Read the model definition and answer for the solid it produces. Units are mm, in the model's axes. A direction names the side the tool comes from. Give positions to 0.01 mm unless a question says otherwise; leave off trailing zeros. Order: outer loops, then holes, each group sorted by start corner. A loop starts at its lowest first (then second) coordinate and runs counter-clockwise, first axis right, second up. Notation, with made-up numbers: (3.5, -5.75) - (41.5, -5.75) arc R15 ccw to (41.5, 9.25) - close; hole circle Ø8 at (67.5, 11). An arc over 180 degrees is marked (long way). Write each question's results on one line, items separated by ' | '. Start each with the question number.
Q1. Find the intervals of material crossed by line 1 along Z through (x, y) = (67, 27); line 2 along Z through (x, y) = (10.5, 12); line 3 along X through (y, z) = (34, 91), in increasing order. Write a range as from..to.
Q2. Flat-ended cylindrical pins translate along their axes: P1, Ø10, axis at y = 9, z = 24, coming from the +X side; P2, Ø6, axis at x = 21, y = 24.5, coming from the -Z side; P3, Ø22.5, axis at x = 49.5, z = 61.5, coming from the -Y side; P4, Ø0.5, axis at y = 20.5, z = 77, coming from the -X side. Find the tip coordinate at first contact, or state that the pin passes through.
Q3. A tool of negligible diameter and unlimited length cuts with its end or side. For faces 4 (the face through (4.88, 33.17, 80.28)), 5 (the face through (38, 36, 15)), 6 (the face through (57.2, 20, 60.4)), 7 (the face through (67, 25, 60)), from which of +Z, -Z, +X, -X, +Y, -Y can it reach the whole face along a straight path? Write none if from no direction.
Q4. Find section C-C on z = 39.5. Give the vertices of the cut face in (x, y) (3 decimals).
Q5. For a pull along X with two mould halves and no side action, classify faces 1 (the face through (17, 0, 30)), 2 (the face through (90.14, 32.675, 50.7)), 3 (the face through (17, 23, 60)) as +X half, -X half, draft (parallel to the pull), parting line (faces both ways), or undercut.
Q6. Find section B-B on x = 71. Give the vertices of the cut face in (y, z).
Q7. Find section D-D on y = 31.5. Give the vertices of the cut face in (x, z).
Q8. Find section A-A on z = 80. Give the vertices of the cut face in (x, y) (3 decimals).
from build123d import *

# Parameters (mm, degrees)
F0_W     = 65
F0_H     = 25
F1_DEPTH = 100
F4_DEPTH = 40
F5_DEPTH = 85
F6_W     = 10
F6_H     = 30
F7_DEPTH = 55
F9_DEPTH = 100.001


with BuildPart() as f1:
    # F0 (on Top) → F1 (new body)
    with BuildSketch(Plane.XY):
        Polygon((0, 45), (0, 0), (35, 0), (35, 20), (35, 45), align=None)
        with Locations((67.5, 32.5)):
            Rectangle(F0_W, F0_H)
    extrude(amount=F1_DEPTH)

    # F2 (on face) → F4 (cut, through all)
    with BuildSketch(Plane.XY.offset(100)):
        Polygon((35, 0), (35, 20), (35, 21), (35, 45), (9.6249980852, 45), (0, 21), (0, 0), align=None)
    extrude(amount=-F4_DEPTH, mode=Mode.SUBTRACT)

    # F2 (on face) → F5 (cut)
    with BuildSketch(Plane.XY.offset(100)):
        Polygon((35, 45), (35, 21), (44.124994427, 45), align=None)
    extrude(amount=-F5_DEPTH, mode=Mode.SUBTRACT)

    # F6 (on face) → F7 (cut)
    with BuildSketch(Plane.YZ.offset(100)):
        with Locations((25, 45)):
            Rectangle(F6_W, F6_H)
    extrude(amount=-F7_DEPTH, mode=Mode.SUBTRACT)

    # F8 (on face) → F9 (cut, through all)
    with BuildSketch(Plane.XY.offset(100)):
        Polygon((100, 20), (100, 45), (80, 20), align=None)
    extrude(amount=-F9_DEPTH, mode=Mode.SUBTRACT)


solid = f1.part
Working result:
1) line 1: 0..30, 60..100 | line 2: 0..60 | line 3: 0..5.21, 39.94..91.2
2) P1: x = 35 | P2: z = 0 | P3: y = 20 | P4: x = 35
3) face 4: +Z, -Y | face 5: +Z, +Y | face 6: +Z, -Z, +X, -Y | face 7: +X, -Y
4) outline: (0, 0) - (35, 0) - (35, 20) - (45, 20) - (45, 30) - (88, 30) - (100, 45) - (44.125, 45) - (35, 21) - (35, 45) - (0, 45) - close
5) face 1: draft | face 2: +X half | face 3: undercut
6) outline: (20, 0) - (45, 0) - (45, 100) - (20, 100) - (20, 60) - (30, 60) - (30, 30) - (20, 30) - close
7) outline: (0, 0) - (89.2, 0) - (89.2, 100) - (38.99, 100) - (38.99, 15) - (35, 15) - (35, 60) - (4.21, 60) - (4.21, 100) - (0, 100) - close
8) outline: (0, 21) - (9.625, 45) - (0, 45) - close; (35, 20) - (80, 20) - (100, 45) - (44.125, 45) - (35, 21) - close
